Solid Edge part; units mm, degrees
sketch "Sketch1" plane through (0, 0, 0) normal (0, -1, 0) x (1, 0, 0)
  circle A0 centre (0, 0) radius 75
extrude "Protrusion1" add sketch "Sketch1" along normal blind 15
sketch "Sketch2" plane through (0, -15, 0) normal (0, -1, 0) x (1, 0, 0)
  circle A0 centre (0, 0) radius 35
extrude "ExtrudedProtrusion_2" add sketch "Sketch2" along normal blind 42.5
sketch "Sketch3" plane through (0, -57.5, 0) normal (0, -1, 0) x (1, 0, 0)
  circle A0 centre (0, 0) radius 15
extrude "ExtrudedCutout_1" cut sketch "Sketch3" against normal blind 241.6449
sketch "Sketch4" plane through (0, -57.5, 0) normal (0, -1, 0) x (1, 0, 0)
  line L0 (-2, 18) -> (2, 18)
  line L1 (2, 18) -> (2, 9.189)
  line L2 (2, 9.189) -> (-2, 9.189)
  line L3 (-2, 9.189) -> (-2, 18)
  dimension "D1" = 2
extrude "ExtrudedCutout_2" cut sketch "Sketch4" against normal blind 185.7022
sketch "Sketch5" plane through (0, -15, 0) normal (0, -1, 0) x (1, 0, 0)
  circle A0 centre (55, 0) radius 7.5
  circle A1 centre (0, -55) radius 7.5
  circle A2 centre (-55, 0) radius 7.5
  circle A3 centre (0, 55) radius 7.5
extrude "ExtrudedCutout_3" cut sketch "Sketch5" against normal blind 96.4879
properties part number "2"
CAD build for the part. Positions are in the model's coordinates, mm. A direction names the side the tool comes from. Coordinates: 2 decimals unless noted, no trailing zeros. Order: outer loops, then holes, each group sorted by start corner. A loop starts at its lowest first (then second) coordinate and runs counter-clockwise, first axis right, second up. Notation, with made-up numbers: (73.25, 26.25) -> (87.25, 26.25) arc R26 cw to (87.25, 59.25) -> close; hole circle Ø3 at (-40, 89). An arc over 180 degrees is marked (long way). Use one line per item in the form item = value. Start each with the question number.
1) Tool access for faces 4 (the flat face through (-32, -15, -16)), 5 (the flat face through (0, -29, 18)), 6 (the flat face through (1, 0, -16)): list every direction of +Z, -Z, +X, -X, +Y, -Y with a clear straight run to the whole face (end or side of a thin tool).
2) Drill centre lines: L1, parallel to Z at x = 0, y = -3; L2, parallel to Z at x = 0, y = -35.5; L3, parallel to Z at x = 5, y = -7.5. Where is each one in solid material? Low to high. Write a range as [from, to].
3) Pull direction X, two halves, no side cores. Call faces 1 (the flat face through (-7, -57.5, -15)), 2 (the cylindrical face through (62.154, -7.605, 2.253)), 3 (the cylindrical face through (-28, -36, 21)): +X half, -X half, draft (parallel to the pull), parting line (faces both ways), or undercut.
4) Band-saw the part on C-C on x = 0. Give the cut face in (y, z), then the cut area to 3 significant figures.
5) Drop flat-ended pins along their axis: pin 1 (17 mm diameter, centred on x = 0, z = 55, fed in from -Y); pin 2 (12 mm diameter, centred on y = -15, z = -22, fed in from +X); pin 3 (1 mm diameter, centred on x = 19, y = -50.5, fed in from +Z); pin 4 (12 mm diameter, centred on x = -55, z = 0, fed in from +Y). Give the stop position or say it passes through.
6) Band-saw the part on B-B on y = -30. Give the cut face in (x, z), then the cut area to 3 significant figures.
7) Band-saw the part on A-A on z = 57.5. Give the cut face in (x, y).
8) Band-saw the part on D-D on x = -55. Give the cut face in (y, z).
Entries:
q1.face_4 = -Y
q1.face_5 = +Y, -Y
q1.face_6 = +Z, -Z, +X, -X, +Y
q2.L1 = [-75, -62.5], [-47.5, -15], [18, 47.5], [62.5, 75]
q2.L2 = [-35, -15], [18, 35]
q2.L3 = [-74.83, -60.59], [-49.41, -14.14], [14.14, 49.41], [60.59, 74.83]
q3.face_1 = draft
q3.face_2 = undercut
q3.face_3 = parting line
q4.outline = (-57.5, -35) -> (-15, -35) -> (-15, -47.5) -> (0, -47.5) -> (0, -15) -> (-57.5, -15) -> close; (-57.5, 18) -> (0, 18) -> (0, 47.5) -> (-15, 47.5) -> (-15, 35) -> (-57.5, 35) -> close; (-15, -75) -> (0, -75) -> (0, -62.5) -> (-15, -62.5) -> close; (-15, 62.5) -> (0, 62.5) -> (0, 75) -> (-15, 75) -> close
q4.area = 2,880 mm2
q5.pin_1 = -15
q5.pin_2 = 73.27
q5.pin_3 = 29.71
q5.pin_4 = through
q6.outline = circle Ø70 at (0, 0); hole (-2, 14.87) arc R15 ccw (long way) to (2, 14.87) -> (2, 18) -> (-2, 18) -> close
q6.area = 3,130 mm2
q7.outline = (-48.15, -15) -> (-7.07, -15) -> (-7.07, 0) -> (-48.15, 0) -> close; (7.07, -15) -> (48.15, -15) -> (48.15, 0) -> (7.07, 0) -> close
q8.outline = (-15, -50.99) -> (0, -50.99) -> (0, -7.5) -> (-15, -7.5) -> close; (-15, 7.5) -> (0, 7.5) -> (0, 50.99) -> (-15, 50.99) -> close
